The figure shows three views and two pictorial views of one solid part (mm, origin at its lowest corner). Answer the questions. A direction names the side the tool comes from. Coordinates: 2 decimals unless noted, no trailing zeros. Order: outer loops, then holes, each group sorted by start corner. A loop starts at its lowest first (then second) coordinate and runs counter-clockwise, first axis right, second up. Notation, with made-up numbers: (70.25, -4) -> (89.25, -4) arc R15 ccw to (89.25, 8) -> close; hole circle Ø6 at (20, -5). An arc over 180 degrees is marked (long way). Return JSON: item names as keys, results as strings.
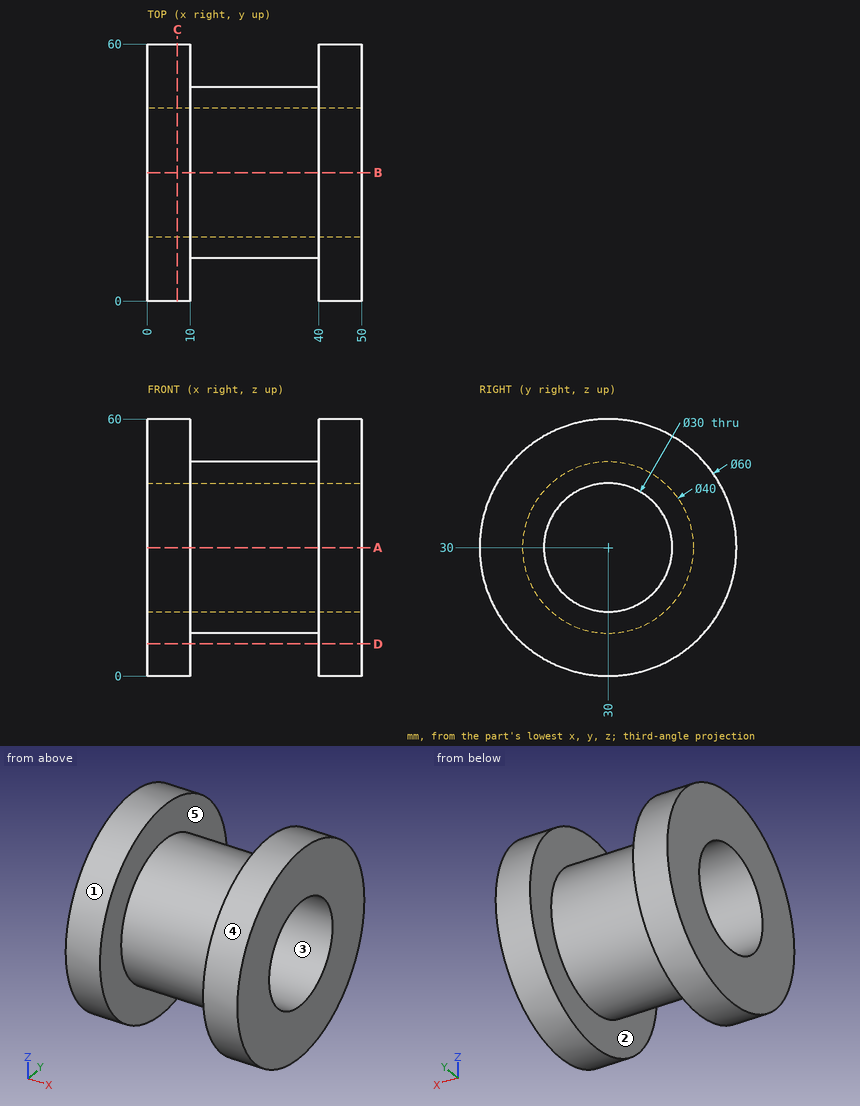
1. Consider line 1 (X direction, y = 6.5, z = 18); line 2 (Z direction, x = 25.5, y = 30); line 3 (Y direction, x = 8, z = 20.5). Determine where each line is inside the solid, lowest interval first. Write a range as from..to.
Answer block:
{"line 1": "x = 0..10, 40..50", "line 2": "z = 10..15, 45..50", "line 3": "y = 1.54..18.39, 41.61..58.46"}
2. The part is cut by section A-A on z = 30. Give the vertices of the cut face in (x, y), and give its area (3 significant figures).
Answer block:
{"outline": "(0, 0) -> (10, 0) -> (10, 10) -> (40, 10) -> (40, 0) -> (50, 0) -> (50, 15) -> (0, 15) -> close; (0, 45) -> (50, 45) -> (50, 60) -> (40, 60) -> (40, 50) -> (10, 50) -> (10, 60) -> (0, 60) -> close", "area": "900 mm2"}
3. Each of these flat-tipped pins is pushed along its axis until it touches: pin 1 Ø6 at (x, z) = (21, 27) entering from -Y; pin 2 Ø4 at (x, z) = (24, 44) entering from -Y; pin 3 Ø1.5 at (y, z) = (9.5, 39) entering from -X; pin 4 Ø10 at (x, y) = (5, 46) entering from -Z. Where does it stop, or does it pass through?
Answer block:
{"pin 1": "stops at y = 10", "pin 2": "stops at y = 14", "pin 3": "stops at x = 0", "pin 4": "stops at z = 2.09"}
4. The part is cut by section C-C on x = 7. Give the vertices of the cut face in (y, z).
Answer block:
{"outline": "circle Ø60 at (30, 30); hole circle Ø30 at (30, 30)"}
5. Determine the mould class of the marked faces 1, 2 and 3 for opening direction Z: pulls with the +Z half, pulls with the -Z half, needs draft (parallel to the pull), parting line crosses it, or undercut.
Answer block:
{"face 1": "parting line crosses it", "face 2": "needs draft", "face 3": "undercut"}
6. For the marked faces 4 and 5, determine the directions among +Z, -Z, +X, -X, +Y, -Y from which every point of the face is accessible in a straight line to the end or side of a thin tool.
Answer block:
{"face 4": "+X, -X", "face 5": "none"}
7. The part is cut by section D-D on z = 7.5. Give the vertices of the cut face in (x, y).
Answer block:
{"outline": "(0, 10.16) -> (10, 10.16) -> (10, 49.84) -> (0, 49.84) -> close; (40, 10.16) -> (50, 10.16) -> (50, 49.84) -> (40, 49.84) -> close"}
